Design review of the part shown in the three views and the two pictorial views. Dimensions are in mm from the part's minimum x, y and z. Give positions to 0.01 mm unless a question says otherwise; leave off trailing zeros. Loops run counter-clockwise (first coordinate to the right, second up) from the corner with the lowest first, then second, coordinate; pieces in that order, holes last. Notation, with made-up numbers: (-21.75, 64.25) - (31.25, 64.25) arc R24 cw to (31.25, 83.25) - close; hole circle Ø4 at (-10, -23). An arc over 180 degrees is marked (long way). Answer in a Markdown table with one row per item.
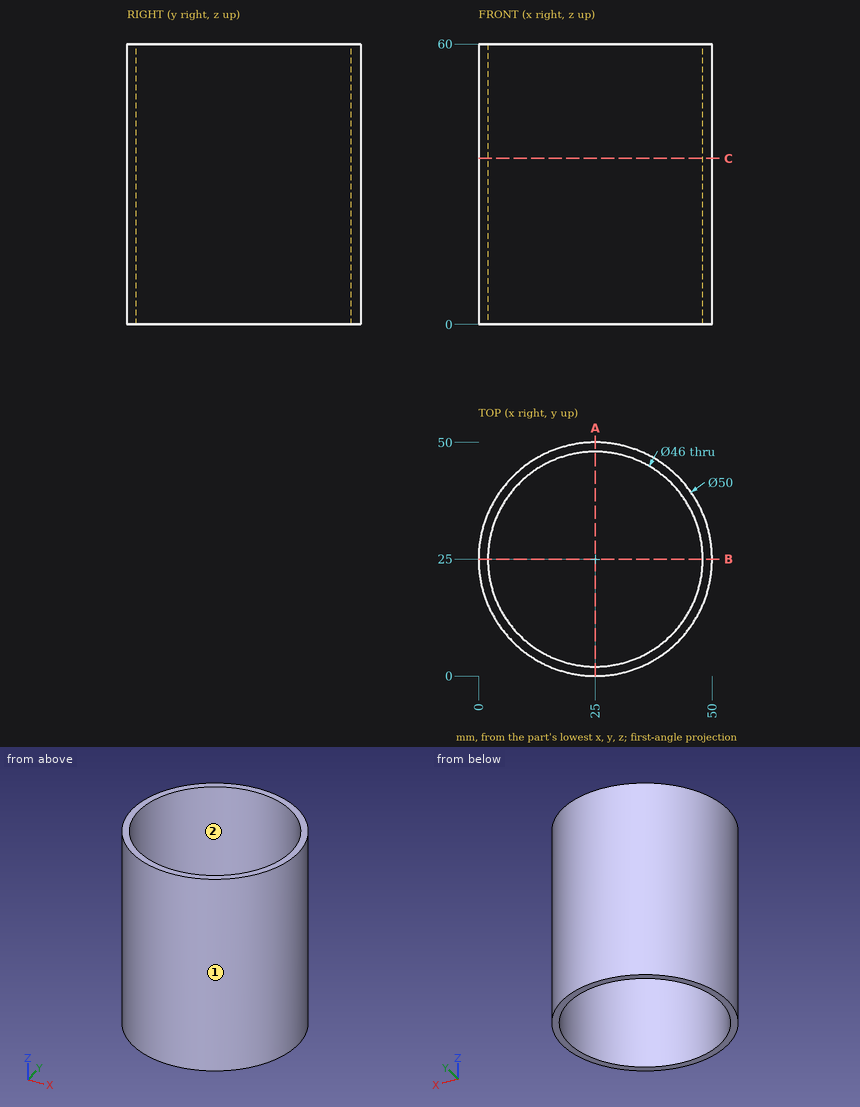
1. Clearance check with flat-ended pins moving along their axes: pin 1 (1.5 mm diameter, centred on x = 20, z = 34, fed in from -Y); pin 2 (8 mm diameter, centred on x = 27.5, z = 49.5, fed in from +Y); pin 3 (5 mm diameter, centred on y = 15, z = 24.5, fed in from +X); pin 4 (2 mm diameter, centred on x = 5, y = 21, fed in from -Z). State where each tip first meets the part, or that it passes through.
Values:
| item | result |
|---|---|
| pin 1 | stops at y = 0.36 |
| pin 2 | stops at y = 50 |
| pin 3 | stops at x = 48.85 |
| pin 4 | passes through |
2. Wall thickness on line 1 (Y direction, x = 25, z = 42.5); line 2 (X direction, y = 33.5, z = 13.5); line 3 (X direction, y = 41, z = 39): over which ranges is each line inside the solid? List them lowest first. Write a range as [from, to].
Values:
| item | result |
|---|---|
| line 1 | y = [0, 2], [48, 50] |
| line 2 | x = [1.49, 3.63], [46.37, 48.51] |
| line 3 | x = [5.79, 8.48], [41.52, 44.21] |
3. We need section A-A, the plane x = 25. Give the boundary of the cut face in (y, z), and give its area (3 significant figures).
Values:
| item | result |
|---|---|
| outline | (0, 0) - (2, 0) - (2, 60) - (0, 60) - close; (48, 0) - (50, 0) - (50, 60) - (48, 60) - close |
| area | 240 mm^2 |
4. Mouldability with a two-part tool opening along X and no side actions: class the marked faces 1 and 2 as released by +X, released by -X, zero draft, split by the parting line, or undercut.
Values:
| item | result |
|---|---|
| face 1 | split by the parting line |
| face 2 | undercut |
5. We need section C-C, the plane z = 35.5. Give the boundary of the cut face in (x, y).
Values:
| item | result |
|---|---|
| outline | circle Ø50 at (25, 25); hole circle Ø46 at (25, 25) |
